from build123d import *

# Parameters (mm, degrees)
F0_W     = 1
F0_H     = 5.5
F0_H_2   = 7.5
F0_W_2   = 2
F0_H_3   = 6.5
F2_DEPTH = 25
F3_DEPTH = 5.5
F4_DEPTH = 5.2


with BuildPart() as f1:
    # F0 (on Front) → F1 (revolve)
    with BuildSketch(Plane.XZ):
        Polygon((9.0724842548, 6.5), (9.0724842548, 0), (10.0724842548, 0), (10.0724842548, 5.5), align=None)
        Polygon((7.0724842548, 6.5), (7.0724842548, 5.5), (7.0724842548, 0), (9.0724842548, 0), (9.0724842548, 6.5), align=None)
        with Locations((6.5724842548, 2.75)):
            Rectangle(F0_W, F0_H)
        with BuildLine():
            Line((-15.9275157452, 6.5), (-15.9275157452, 0))
            Line((-15.9275157452, 0), (-12.9275157452, 0))
            ThreePointArc((-12.9275157452, 0), (-12.1952826981, 1.767766953), (-10.4275157452, 2.5))
            Line((-10.4275157452, 2.5), (0.5724842548, 2.5))
            ThreePointArc((0.5724842548, 2.5), (2.3402512078, 1.767766953), (3.0724842548, 0))
            Line((3.0724842548, 0), (6.0724842548, 0))
            Line((6.0724842548, 0), (6.0724842548, 5.5))
            Line((6.0724842548, 5.5), (6.0724842548, 6.5))
            Line((6.0724842548, 6.5), (-15.9275157452, 6.5))
        make_face()
        with BuildLine():
            ThreePointArc((-10.4275157452, 2.5), (-12.1952826981, 1.767766953), (-12.9275157452, 0))
            Line((-12.9275157452, 0), (3.0724842548, 0))
            ThreePointArc((3.0724842548, 0), (2.3402512078, 1.767766953), (0.5724842548, 2.5))
            Line((0.5724842548, 2.5), (-10.4275157452, 2.5))
        make_face()
        Polygon((-24.9275157452, 7.5), (-24.9275157452, 0), (-15.9275157452, 0), (-15.9275157452, 6.5), (-15.9275157452, 7.5), align=None)
        with Locations((-25.4275157452, 3.75)):
            Rectangle(F0_W, F0_H_2)
        Polygon((-27.9275157452, 8.5), (-27.9275157452, 7.5), (-27.9275157452, 0), (-25.9275157452, 0), (-25.9275157452, 7.5), (-25.9275157452, 8.5), align=None)
        with BuildLine():
            Line((-27.9275157452, 7.5), (-48.9275157452, 7.5))
            Line((-48.9275157452, 7.5), (-48.9275157452, 6.5))
            Line((-48.9275157452, 6.5), (-48.9275157452, 0))
            Line((-48.9275157452, 0), (-46.4275157452, 0))
            ThreePointArc((-46.4275157452, 0), (-45.6952826981, 1.767766953), (-43.9275157452, 2.5))
            Line((-43.9275157452, 2.5), (-32.9275157452, 2.5))
            ThreePointArc((-32.9275157452, 2.5), (-31.1597487922, 1.767766953), (-30.4275157452, 0))
            Line((-30.4275157452, 0), (-27.9275157452, 0))
            Line((-27.9275157452, 0), (-27.9275157452, 7.5))
        make_face()
        with BuildLine():
            ThreePointArc((-43.9275157452, 2.5), (-45.6952826981, 1.767766953), (-46.4275157452, 0))
            Line((-46.4275157452, 0), (-30.4275157452, 0))
            ThreePointArc((-30.4275157452, 0), (-31.1597487922, 1.767766953), (-32.9275157452, 2.5))
            Line((-32.9275157452, 2.5), (-43.9275157452, 2.5))
        make_face()
        with Locations((-49.9275157452, 3.25)):
            Rectangle(F0_W_2, F0_H_3)
        Polygon((-50.9275157452, 0), (-50.9275157452, 6.5), (-50.9275157452, 7.5), (-60.9275157452, 7.5), (-60.9275157452, 0), align=None)
        Polygon((-61.9275157452, 0), (-60.9275157452, 0), (-60.9275157452, 7.5), (-61.9275157452, 6.5), align=None)
    revolve(axis=Axis((-25.9275157452, 0, 0), (1, 0, 0)))

    # F0 (on Front) → F2 (cut)
    with BuildSketch(Plane.XZ):
        with BuildLine():
            Line((-30.4275157452, 0), (-46.4275157452, 0))
            ThreePointArc((-46.4275157452, 0), (-45.6952826981, -1.767766953), (-43.9275157452, -2.5))
            Line((-43.9275157452, -2.5), (-32.9275157452, -2.5))
            ThreePointArc((-32.9275157452, -2.5), (-31.1597487922, -1.767766953), (-30.4275157452, 0))
        make_face()
        with BuildLine():
            ThreePointArc((-43.9275157452, 2.5), (-45.6952826981, 1.767766953), (-46.4275157452, 0))
            Line((-46.4275157452, 0), (-30.4275157452, 0))
            ThreePointArc((-30.4275157452, 0), (-31.1597487922, 1.767766953), (-32.9275157452, 2.5))
            Line((-32.9275157452, 2.5), (-43.9275157452, 2.5))
        make_face()
        with BuildLine():
            ThreePointArc((-10.4275157452, 2.5), (-12.1952826981, 1.767766953), (-12.9275157452, 0))
            Line((-12.9275157452, 0), (3.0724842548, 0))
            ThreePointArc((3.0724842548, 0), (2.3402512078, 1.767766953), (0.5724842548, 2.5))
            Line((0.5724842548, 2.5), (-10.4275157452, 2.5))
        make_face()
        with BuildLine():
            Line((3.0724842548, 0), (-12.9275157452, 0))
            ThreePointArc((-12.9275157452, 0), (-12.1952826981, -1.767766953), (-10.4275157452, -2.5))
            Line((-10.4275157452, -2.5), (0.5724842548, -2.5))
            ThreePointArc((0.5724842548, -2.5), (2.3402512078, -1.767766953), (3.0724842548, 0))
        make_face()
    extrude(amount=F2_DEPTH, mode=Mode.SUBTRACT)

    # F3 (add): a face of the model
    f3_faces = [f1.faces().sort_by_distance(p)[0] for p in [
        (-38.4275157452, 0, 0),
    ]]
    extrude(f3_faces, amount=F3_DEPTH)

    # F4 (add): a face of the model
    f4_faces = [f1.faces().sort_by_distance(p)[0] for p in [
        (-4.9275157452, 0, 0),
    ]]
    extrude(f4_faces, amount=F4_DEPTH)


solid = f1.part
Build history of the part. All positions in model axes, mm. A direction names the side the tool comes from. Give positions to 0.01 mm unless a question says otherwise; leave off trailing zeros. Write each loop counter-clockwise with the first axis right and the second up, starting at its lowest first coordinate (ties: lowest second). Pieces come first, ordered by that corner, then holes. Notation, with made-up numbers: (52, -29) - (111, -29) arc R35 ccw to (111, 4) - close; hole circle Ø3 at (50.25, 50.5). An arc over 180 degrees is marked (long way). Use one line per item in the form item = value. Start each with the question number.
1. 3-axis set-ups, long thin cutter, end or side, ignore diameter. For faces 5 (the face through (7.072, -3, -5)), 6 (the face through (-5, -5.2, 0)), 7 (the face through (-26.942, -7.167, 4.57)), 8 (the face through (-55.998, -0.33, -7.493)), 9 (the face through (-20.998, -0.33, -7.493)): which of +Z, -Z, +X, -X, +Y, -Y reach the whole face in a straight line?
2. Probe line 1 (Y direction, x = -44.5, z = -3.75); line 2 (X direction, y = -4, z = -4.5). List the from-to ranges inside material, lowest first. Write a range as [from, to].
3. Band-saw the part on B-B on x = -57. Write the cut outline in (y, z).
4. Band-saw the part on A-A on x = -7.5. Write the cut outline in (y, z), plus the area to 3 significant figures.
5. Drop flat-ended pins along their axis: pin 1 Ø1.5 at (x, z) = (-42.5, 0) entering from -Y; pin 2 Ø5 at (x, z) = (-46.5, 5.5) entering from +Y; pin 3 Ø1 at (x, y) = (-48.5, 2.5) entering from +Z. Give the stop position or say it passes through.
6. Two-plate mould, pull along Z, no slides. Class faces 1 (the face through (-39, -6, -2.5)), 2 (the face through (-49.914, 3.955, -5.158)), 3 (the face through (-38, -6, 2.5)), 4 (the face through (-61.928, 0, 0)): released by +Z, released by -Z, zero draft, split by the parting line, or undercut.
Conclusion:
q1.face_5 = none
q1.face_6 = -Y
q1.face_7 = +X, -X
q1.face_8 = -X
q1.face_9 = +X
q2.line_1 = [-6.5, 6.5]
q2.line_2 = [-61.93, 6.07], [7.07, 9.55]
q3.outline = circle Ø15 at (0, 0)
q4.outline = (-6, -2.5) arc R6.5 ccw (long way) to (-6, 2.5) - (-5.2, 2.5) - (-5.2, -2.5) - close
q4.area = 127 mm²
q5.pin_1 = -5.5
q5.pin_2 = 6.87
q5.pin_3 = 7.23
q6.face_1 = undercut
q6.face_2 = split by the parting line
q6.face_3 = undercut
q6.face_4 = zero draft
